Input: dimensioned drawing with shaded views. Units: mm. Origin: part minimum x, y, z. Give positions to 0.01 mm unless a question says otherwise; leave off trailing zeros. Loops run counter-clockwise (first coordinate to the right, second up) from the corner with the lowest first, then second, coordinate; pieces in that order, holes last.
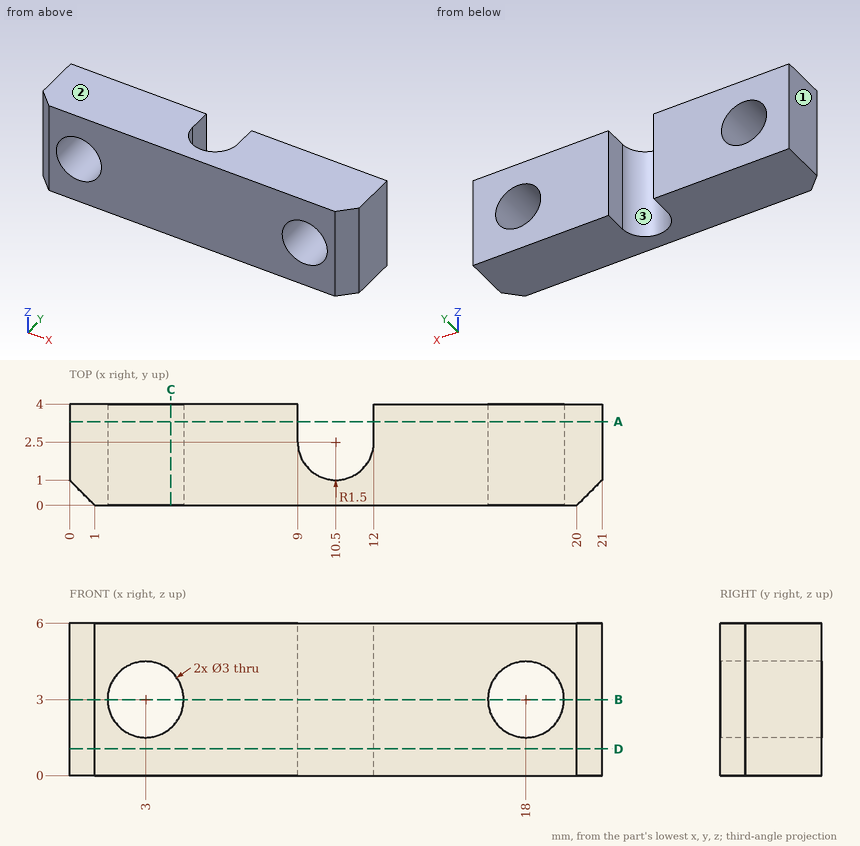
(1) Section D-D, the plane z = 1.05. Return the cut outline in (x, y), then the cut area to 3 significant figures.
A:
outline: (0, 1) - (1, 0) - (20, 0) - (21, 1) - (21, 4) - (12, 4) - (12, 2.5) arc R1.5 cw to (9, 2.5) - (9, 4) - (0, 4) - close
area: 75.0 mm2
(2) Ray query, line 1 along Z through (x, y) = (3, 1.65); line 2 along X through (y, z) = (2.95, 0.9); line 3 along X through (y, z) = (2.9, 3). Return the intervals inside material, ascending.
A:
line 1: z = 0 to 1.5, 4.5 to 6
line 2: x = 0 to 9, 12 to 21
line 3: x = 0 to 1.5, 4.5 to 9, 12 to 16.5, 19.5 to 21
(3) Section C-C, the plane x = 4. Return the cut outline in (y, z).
A:
outline: (0, 0) - (4, 0) - (4, 1.88) - (0, 1.88) - close; (0, 4.12) - (4, 4.12) - (4, 6) - (0, 6) - close
(4) Section B-B, the plane z = 3. Return the cut outline in (x, y), then the cut area to 3 significant figures.
A:
outline: (0, 1) - (1, 0) - (1.5, 0) - (1.5, 4) - (0, 4) - close; (4.5, 0) - (16.5, 0) - (16.5, 4) - (12, 4) - (12, 2.5) arc R1.5 cw to (9, 2.5) - (9, 4) - (4.5, 4) - close; (19.5, 0) - (20, 0) - (21, 1) - (21, 4) - (19.5, 4) - close
area: 51.0 mm2
(5) Section A-A, the plane y = 3.3. Return the cut outline in (x, z), then the cut area to 3 significant figures.
A:
outline: (0, 0) - (9, 0) - (9, 6) - (0, 6) - close; (12, 0) - (21, 0) - (21, 6) - (12, 6) - close; hole circle Ø3 at (3, 3); hole circle Ø3 at (18, 3)
area: 93.9 mm2
(6) Mould query, pull axis X, two halves, no side actions, for the marked faces 1, 2 and 3. Classes: pulls with the +X half, pulls with the -X half, needs draft (parallel to the pull), parting line crosses it, or undercut.
A:
face 1: pulls with the -X half
face 2: needs draft
face 3: undercut
